Here's the drawing with two shaded views (mm, measured from the low corner). I have some questions. A direction names the side the tool comes from. Give positions to 0.01 mm unless a question says otherwise; leave off trailing zeros. Loops run counter-clockwise (first coordinate to the right, second up) from the corner with the lowest first, then second, coordinate; pieces in that order, holes last. Notation, with made-up numbers: M 12,21 L 66,21 A24 ccw 66,51 Z; hole C 16,43.5 d8. An arc over 180 degrees is marked long. Answer in a Markdown table with one row per item. Add a question column.
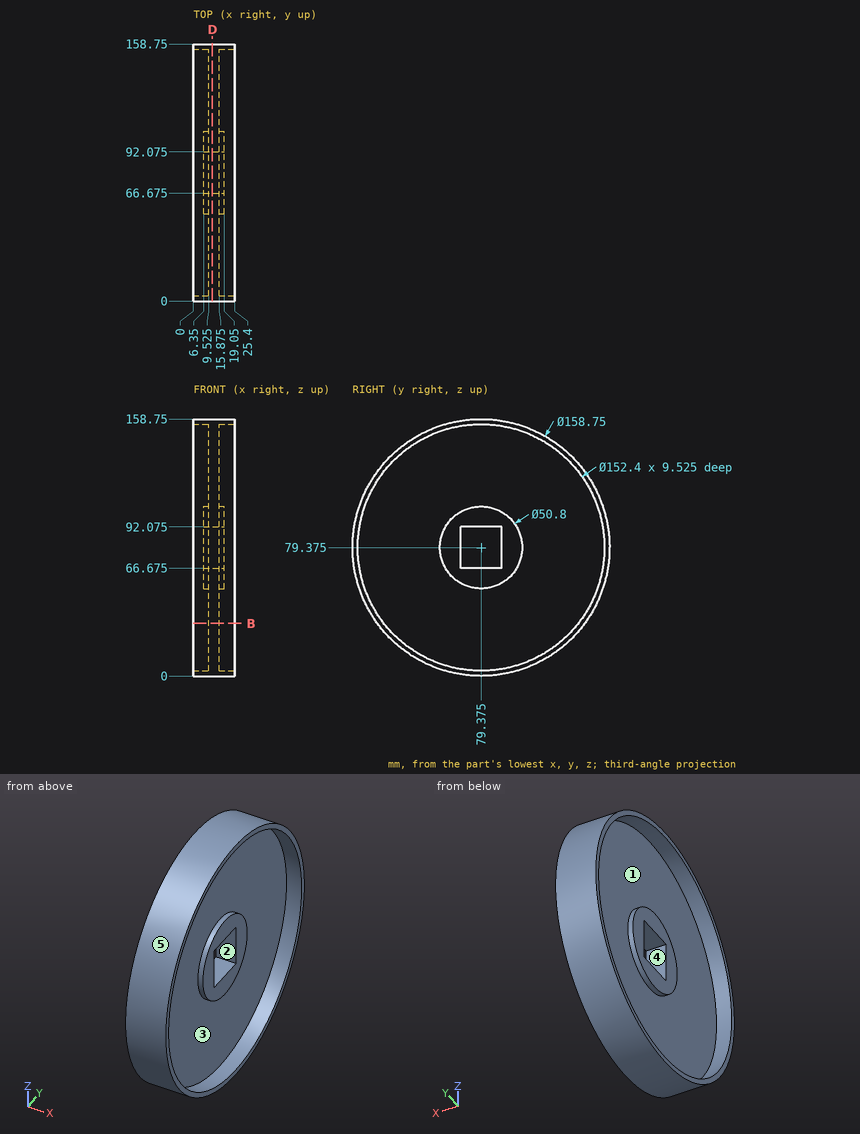
Item 1: If we mould it in two halves opening along Y, with no side actions, what happens to the marked faces 4 and 5? For each: +Y half, -Y half, draft (parallel to the pull), parting line (faces both ways), or undercut.
Item 2: I need wall thicknesses on L1, parallel to Z at x = 16.25, y = 90.5 (1 decimal); L2, parallel to X at y = 103.5, z = 75; L3, parallel to Y at x = 16.5, z = 92.5. Which ranges of each line are inside material? Lowest first, please.
Item 3: Suppose I cut it at B-B (z = 32.5). List the corners of the cut face in (x, y) for me (3 decimals).
Item 4: For the marked faces 1, 2 and 3, which set-ups out of +Z, -Z, +X, -X, +Y, -Y let a thin tool reach every point of the face, with its end or its side?
Item 5: Suppose I cut it at D-D (x = 11.75). List the corners of the cut face in (y, z) for me (3 decimals), then the cut area to 3 significant figures.
Item 6: For P1, Ø10, axis at x = 15.5, z = 82.5, coming from the -Y side; P2, Ø6, axis at y = 59.5, z = 50.5, coming from the +X side (3 decimals); P3, Ø3, axis at x = 22.5, y = 139.5, coming from the +Z side, each with a flat end and sliding along its axis, tell me the tip position at first contact or that it passes through.
Values found:
| question | item | result |
|---|---|---|
| 1 | face 4 | undercut |
| 1 | face 5 | parting line |
| 2 | L1 | 0.8 to 4, 56.5 to 66.7, 92.1 to 102.2, 154.8 to 158 |
| 2 | L2 | 6.35 to 19.05 |
| 2 | L3 | 1.09 to 4.31, 57.63 to 101.12, 154.44 to 157.66 |
| 3 | outline | M 0,15.319 L 25.4,15.319 L 25.4,19.299 L 15.875,19.299 L 15.875,139.451 L 25.4,139.451 L 25.4,143.431 L 0,143.431 L 0,139.451 L 9.525,139.451 L 9.525,19.299 L 0,19.299 Z |
| 4 | face 1 | -X |
| 4 | face 2 | +X, -X |
| 4 | face 3 | +X |
| 5 | outline | C 79.375,79.375 d158.75; hole M 66.675,66.675 L 92.075,66.675 L 92.075,92.075 L 66.675,92.075 Z |
| 5 | area | 19,100 mm² |
| 6 | P1 | y = 0 |
| 6 | P2 | x = 15.875 |
| 6 | P3 | z = 132.89 |
